from build123d import *

# Parameters (mm, degrees)
SKETCH1_W           = 60
SKETCH1_H           = 6.32
BOSS_EXTRUDE1_DEPTH = 10.64
SKETCH2_R           = 5
CUT_EXTRUDE1_DEPTH  = 64.974845056
SKETCH3_W           = 6.32
SKETCH3_H           = 21.28
BOSS_EXTRUDE2_DEPTH = 21.5
SKETCH4_W           = 6.32
SKETCH4_H           = 21.28
BOSS_EXTRUDE3_DEPTH = 21.5
SKETCH5_W           = 8
SKETCH5_H           = 21.28
BOSS_EXTRUDE6_DEPTH = 84.33
SKETCH6_W           = 8
SKETCH6_H           = 21.291954735
BOSS_EXTRUDE7_DEPTH = 84.33
SKETCH7_W           = 6.32
SKETCH7_H           = 21.291954735
BOSS_EXTRUDE8_DEPTH = 95
SKETCH9_R           = 5
CUT_EXTRUDE2_DEPTH  = 120.193734049
SKETCH10_R          = 2.22
CUT_EXTRUDE3_DEPTH  = 123.364768784
FILLET1_R           = 3
SKETCH13_R          = 3.175
CUT_EXTRUDE4_DEPTH  = 123.364768784
SKETCH17_W          = 12.954
SKETCH17_H          = 7.031857888
CUT_EXTRUDE7_DEPTH  = 12.7
CUT_EXTRUDE8_REACH  = 124.365
SKETCH18_W          = 6.477
SKETCH18_H          = 8.58
SKETCH19_R          = 3.175
CUT_EXTRUDE9_DEPTH  = 134.544049061


with BuildPart() as part:
    # Sketch1 → Boss-Extrude1 (new, symmetric)
    with BuildSketch(Plane(origin=(0, 0, 0), x_dir=(1, 0, 0), z_dir=(0, 1, 0))):
        with Locations((30, -3.16)):
            Rectangle(SKETCH1_W, SKETCH1_H)
    extrude(amount=BOSS_EXTRUDE1_DEPTH, both=True)

    # Sketch2 → Cut-Extrude1 (cut, through all)
    with BuildSketch(Plane(origin=(0, 10.64, 0), x_dir=(1, 0, 0), z_dir=(0, 1, 0))):
        with Locations((7.21, 1.25)):
            Circle(SKETCH2_R)
        with Locations((52.79, 1.25)):
            Circle(SKETCH2_R)
    extrude(amount=-CUT_EXTRUDE1_DEPTH, mode=Mode.SUBTRACT)

    # Sketch3 → Boss-Extrude2 (add)
    with BuildSketch(Plane(origin=(60, 0, 0), x_dir=(0, 0, -1), z_dir=(1, 0, 0))):
        with Locations((-3.16, 0)):
            Rectangle(SKETCH3_W, SKETCH3_H)
    extrude(amount=BOSS_EXTRUDE2_DEPTH)

    # Sketch4 → Boss-Extrude3 (add)
    with BuildSketch(Plane.ZY):
        with Locations((3.16, 0)):
            Rectangle(SKETCH4_W, SKETCH4_H)
    extrude(amount=BOSS_EXTRUDE3_DEPTH)

    # Sketch5 → Boss-Extrude6 (add)
    with BuildSketch(Plane(origin=(0, 0, 0), x_dir=(-1, 0, 0), z_dir=(0, 0, -1))):
        with Locations((17.5, 0)):
            Rectangle(SKETCH5_W, SKETCH5_H)
    extrude(amount=BOSS_EXTRUDE6_DEPTH)

    # Sketch6 → Boss-Extrude7 (add)
    with BuildSketch(Plane(origin=(0, 0, 0), x_dir=(-1, 0, 0), z_dir=(0, 0, -1))):
        with Locations((-77.5, -0.005977367)):
            Rectangle(SKETCH6_W, SKETCH6_H)
    extrude(amount=BOSS_EXTRUDE7_DEPTH)

    # Sketch7 → Boss-Extrude8 (add, through all)
    with BuildSketch(Plane.ZY.offset(-73.5)):
        with Locations((-81.17, -0.005977367)):
            Rectangle(SKETCH7_W, SKETCH7_H)
    extrude(amount=BOSS_EXTRUDE8_DEPTH)

    # Sketch9 → Cut-Extrude2 (cut, through all)
    with BuildSketch(Plane(origin=(0, 10.64, 0), x_dir=(1, 0, 0), z_dir=(0, 1, 0))):
        with Locations((7.21, 76.76)):
            Circle(SKETCH9_R)
        with Locations((52.79, 76.76)):
            Circle(SKETCH9_R)
    extrude(amount=-CUT_EXTRUDE2_DEPTH, mode=Mode.SUBTRACT)

    # Sketch10 → Cut-Extrude3 (cut, through all)
    with BuildSketch(Plane(origin=(0, 0, -84.33), x_dir=(-1, 0, 0), z_dir=(0, 0, -1))):
        with Locations((-62.631229183, 0.005)):
            Circle(SKETCH10_R)
        with Locations((2.631229183, 0.005)):
            Circle(SKETCH10_R)
    extrude(amount=-CUT_EXTRUDE3_DEPTH, mode=Mode.SUBTRACT)

    # Fillet1
    fillet1_edges = [part.edges().sort_by_distance(p)[0] for p in [
        (81.5, 0, 6.32),
        (-21.5, 0, 6.32),
        (-13.5, 0, 0),
        (-21.5, -0.005977367, -84.33),
        (73.5, 0, 0),
        (81.5, -0.005977367, -84.33),
        (-13.5, 0, -78.01),
        (73.5, -0.005977367, -78.01),
    ]]
    fillet(fillet1_edges, radius=FILLET1_R)

    # Sketch13 → Cut-Extrude4 (cut, through all)
    with BuildSketch(Plane(origin=(0, 0, -84.33), x_dir=(-1, 0, 0), z_dir=(0, 0, -1))):
        with Locations((-30, 0.005)):
            Circle(SKETCH13_R)
    extrude(amount=-CUT_EXTRUDE4_DEPTH, mode=Mode.SUBTRACT)

    # Sketch17 → Cut-Extrude7 (cut, symmetric)
    with BuildSketch(Plane(origin=(0, 10.64, 0), x_dir=(1, 0, 0), z_dir=(0, 1, 0))):
        with Locations((19.173393665, -2.929761462)):
            Rectangle(SKETCH17_W, SKETCH17_H)
    extrude(amount=CUT_EXTRUDE7_DEPTH, both=True, mode=Mode.SUBTRACT)

    # Sketch18 → Cut-Extrude8 (cut, up to next)
    with BuildSketch(Plane.XY.offset(6.32), mode=Mode.PRIVATE) as cut_extrude8_sk1:
        with Locations((22.411893665, -6.35)):
            Rectangle(SKETCH18_W, SKETCH18_H)
    cut_extrude8_tool1 = extrude(cut_extrude8_sk1.sketch, amount=-CUT_EXTRUDE8_REACH, mode=Mode.PRIVATE) & part.part
    add(cut_extrude8_tool1.solids().sort_by_distance((22.411894, -6.35, 6.32))[0], mode=Mode.SUBTRACT)

    # Sketch19 → Cut-Extrude9 (cut, through all)
    with BuildSketch(Plane.ZY.offset(21.5)):
        with Locations((-39.005, 0)):
            Circle(SKETCH19_R)
    extrude(amount=-CUT_EXTRUDE9_DEPTH, mode=Mode.SUBTRACT)


solid = part.part
Design review of the part built by this model. Coordinates are the model's own, in mm. A direction names the side the tool comes from. Give positions to 0.01 mm unless a question says otherwise; leave off trailing zeros. Order: outer loops, then holes, each group sorted by start corner. A loop starts at its lowest first (then second) coordinate and runs counter-clockwise, first axis right, second up. Notation, with made-up numbers: (-28, -31.75) - (12, -31.75) arc R19 cw to (12, -15.75) - close; hole circle Ø6 at (1.25, -10.75). An arc over 180 degrees is marked (long way). Use CSV: the item, a comma, the result in double quotes. Start each with the question number.
Q1. Take a section at D-D (y = -7). State the section outline as (x, z) points, and give its area (3 significant figures).
Q2. For P1, Ø5, axis at y = -6.5, z = 4.5, coming from the +X side; P2, Ø4, axis at x = -2.63, y = 0, coming from the +Z side, all flat-tipped, find the tip position at first contact; note any pin that passes through.
Q3. Machinability: for faces 1 (the face through (25.65, 0, 3)), 2 (the face through (73.5, -3, -37)), 3 (the face through (52, 0, 6.32)), which of the approach directions +Z, -Z, +X, -X, +Y, -Y give a long, thin tool a straight path to every point of the face, cutting with its end or side? Answer none if there is none.
Q4. For line 1 (X direction, y = -4, z = -73); line 2 (Z direction, x = 70, y = 6.5); line 3 (Y direction, x = 30, z = -82), list the stretches that pass through material, from the lowest coordinate up.
Q5. Take a section at B-B (x = 45.5). State the section outline as (y, z) points, and give its area (3 significant figures).
Q6. Take a section at A-A (z = -28). State the section outline as (x, y) points.
Q7. Draft analysis for pull direction X (two halves, no side actions). For faces 4 (the face through (-21.5, 5, -40)), 5 (the face through (64.85, 0.1, 3.12)), 6 (the face through (54, -10.64, 4)), state which applies: pulls with the +X half, pulls with the -X half, needs draft (parallel to the pull), parting line crosses it, or undercut.
Q8. Take a section at C-C (x = 30). State the section outline as (y, z) points, and give its area (3 significant figures).
Calculated:
1,outline,"(-21.5, -81.33) arc R3 ccw to (-18.5, -84.33) - (78.5, -84.33) arc R3 ccw to (81.5, -81.33) - (81.5, 3.32) arc R3 ccw to (78.5, 6.32) - (25.65, 6.32) - (25.65, 0) - (47.95, 0) arc R5 cw to (57.63, 0) - (70.5, 0) arc R3 cw to (73.5, -3) - (73.5, -75.01) arc R3 cw to (70.5, -78.01) - (57.63, -78.01) arc R5 cw to (47.95, -78.01) - (12.05, -78.01) arc R5 cw to (2.37, -78.01) - (-10.5, -78.01) arc R3 cw to (-13.5, -75.01) - (-13.5, -3) arc R3 cw to (-10.5, 0) - (2.37, 0) arc R5 cw to (12.05, 0) - (19.17, 0) - (19.17, 6.32) - (-18.5, 6.32) arc R3 ccw to (-21.5, 3.32) - close"
1,area,"2,400 mm²"
2,P1,"stops at x = 81.5"
2,P2,"passes through"
3,face 1,"+Z, +Y, -Y"
3,face 2,"+Y, -Y"
3,face 3,"+Z, +X, -X, +Y, -Y"
4,line 1,"x = -21.5 to -13.5, 73.5 to 81.5"
4,line 2,"z = -84.33 to -78.01, 0 to 6.32"
4,line 3,"y = -10.65 to -3.17, 3.18 to 10.64"
5,outline,"(-10.65, -84.33) - (10.64, -84.33) - (10.64, -78.01) - (-10.65, -78.01) - close; (-10.64, 0) - (10.64, 0) - (10.64, 6.32) - (-10.64, 6.32) - close"
5,area,"269 mm²"
6,outline,"(-21.5, -10.64) - (-13.5, -10.64) - (-13.5, 10.64) - (-21.5, 10.64) - close; (73.5, -10.65) - (81.5, -10.65) - (81.5, 10.64) - (73.5, 10.64) - close"
7,face 4,"pulls with the -X half"
7,face 5,"undercut"
7,face 6,"needs draft"
8,outline,"(-10.65, -84.33) - (-3.17, -84.33) - (-3.17, -78.01) - (-10.65, -78.01) - close; (-10.64, 0) - (-3.17, 0) - (-3.17, 6.32) - (-10.64, 6.32) - close; (3.18, -84.33) - (10.64, -84.33) - (10.64, -78.01) - (3.18, -78.01) - close; (3.18, 0) - (10.64, 0) - (10.64, 6.32) - (3.18, 6.32) - close"
8,area,"189 mm²"
